from build123d import *

# Parameters (mm, degrees)
SKETCH1_W           = 38.1
SKETCH1_H           = 44.45
BOSS_EXTRUDE1_DEPTH = 25.4


with BuildPart() as part:
    # Sketch1 → Boss-Extrude1 (new body)
    with BuildSketch(Plane.XY):
        with Locations((19.05, -22.225)):
            Rectangle(SKETCH1_W, SKETCH1_H)
        Polygon((38.1, -596.9), (0, -44.45), (38.1, -44.45), (63.5, -596.9), align=None)
    extrude(amount=BOSS_EXTRUDE1_DEPTH)


solid = part.part
Verification items for the finished model (mm, model axes). A direction names the side the tool comes from. Round coordinates to 2 decimals unless told otherwise and drop trailing zeros. Loops run counter-clockwise (first coordinate to the right, second up) from the corner with the lowest first, then second, coordinate; pieces in that order, holes last. Notation, with made-up numbers: (-3.75, -36) - (13.25, -36) arc R19 cw to (13.25, -13) - close; hole circle Ø5 at (-37, -25). An arc over 180 degrees is marked (long way). Use a Markdown table: item, result. Add a question column.
1. Gauge pin test, flat ends, axial feed: pin 1 (4 mm diameter, centred on y = -335.5, z = 20, fed in from -X); pin 2 (1 mm diameter, centred on y = -167, z = 7, fed in from +X); pin 3 (3 mm diameter, centred on y = -113, z = 9.5, fed in from +X); pin 4 (1 mm diameter, centred on x = 6.5, z = 14.5, fed in from +Y). Record the tip position at first contact, or that the pin passes through.
2. Section check B-B, the plane x = 16. Record the boundary of the cut face in (y, z).
3. Section check A-A, the plane z = 11.5. Record the boundary of the cut face in (x, y), plus the area to 3 significant figures.
4. Thickness scan on probe 1 along X at (y, z) = (-139.5, 9.5); probe 2 along X at (y, z) = (-379, 16.5). Record the ranges inside material, lowest first. Write a range as [from, to].
5. Access from +Z, -Z, +X, -X, +Y, -Y to the whole of each face (thin tool, end or side, straight path). Record for faces 1 (the face through (38.1, -23, 13)), 2 (the face through (31, -294, 0)).
6. Section check C-C, the plane y = -74.5. Record the boundary of the cut face in (x, z).
7. Release check for a two-part mould opening along Y. For faces 3 (the face through (31, -294, 25.4)), 4 (the face through (51, -596.9, 13)), 5 (the face through (50.622, -316.808, 12.522)) record: released by +Y, released by -Y, zero draft, split by the parting line, or undercut.
Checks:
| question | item | result |
|---|---|---|
| 1 | pin 1 | stops at x = 19.93 |
| 1 | pin 2 | stops at x = 43.76 |
| 1 | pin 3 | stops at x = 41.32 |
| 1 | pin 4 | stops at y = 0 |
| 2 | outline | (-276.45, 0) - (0, 0) - (0, 25.4) - (-276.45, 25.4) - close |
| 3 | outline | (0, -44.45) - (38.1, -596.9) - (63.5, -596.9) - (38.1, -44.45) - (38.1, 0) - (0, 0) - close |
| 3 | area | 19,200 mm^2 |
| 4 | probe 1 | x = [6.56, 42.47] |
| 4 | probe 2 | x = [23.07, 53.48] |
| 5 | face 1 | +Z, -Z, +X, +Y |
| 5 | face 2 | -Z, +X, -X, +Y, -Y |
| 6 | outline | (2.07, 0) - (39.48, 0) - (39.48, 25.4) - (2.07, 25.4) - close |
| 7 | face 3 | zero draft |
| 7 | face 4 | released by -Y |
| 7 | face 5 | released by +Y |
